Autodesk Inventor part; units mm, degrees
ref_plane "YZ Plane" through (0, 0, 0) normal (1, 0, 0) x (0, 1, 0)
ref_plane "XZ Plane" through (0, 0, 0) normal (0, 1, 0) x (-1, 0, 0)
ref_plane "XY Plane" through (0, 0, 0) normal (0, 0, 1) x (1, 0, 0)
sketch "Sketch1" plane through (0, 0, 0) normal (0, 1, 0) x (-1, 0, 0)
  line L0 (85, -50) -> (65, -50)
  line L1 (-85, -50) -> (-85, 0)
  line L2 (-85, 0) -> (85, 0)
  line L3 (85, 0) -> (85, -50)
  line L4 (85, -50) -> (-85, 0) construction
  line L5 (-85, -50) -> (85, 0) construction
  arc A0 (65, -50) -> (-65, -50) centre (0, -126.0208) ccw
  line L6 (65, -50) -> (-65, -50) construction
  line L7 (-65, -50) -> (-85, -50)
  line L8 (65, -28.5948) -> (65, -14)
  line L9 (63, -12) -> (30.2021, -12)
  arc A1 (61.914, -30.2742) -> (29.6815, -15.931) centre (0, -126.0208) ccw
  line L10 (0, 0) -> (0, -25)
  arc A2 (30.2021, -12) -> (29.6815, -15.931) centre (30.2021, -14) ccw
  arc A3 (65, -14) -> (63, -12) centre (63, -14) ccw
  arc A4 (61.914, -30.2742) -> (65, -28.5948) centre (63, -28.5948) ccw
  line L11 (-65, -28.5948) -> (-65, -14)
  line L12 (-63, -12) -> (-30.2021, -12)
  arc A5 (-29.6815, -15.931) -> (-61.914, -30.2742) centre (0, -126.0208) ccw
  arc A6 (-29.6815, -15.931) -> (-30.2021, -12) centre (-30.2021, -14) ccw
  arc A7 (-63, -12) -> (-65, -14) centre (-63, -14) ccw
  arc A8 (-65, -28.5948) -> (-61.914, -30.2742) centre (-63, -28.5948) ccw
  point P0 (0, -25)
  point P1 (0, -25)
  point P2 (65, -32.3419)
  point P3 (0, -12)
  dimension "d0" = 170
  dimension "d1" = 50
  dimension "d2" = 26
  dimension "d3" = 20
  dimension "d4" = 12
  dimension "d5" = 20
  dimension "d6" = 2
extrude "Extrusion1" add sketch "Sketch1" along normal mid plane 3.175
sketch "Sketch2" plane through (0, 1.5875, 0) normal (0, 1, 0) x (1, 0, 0)
  line L0 (-85, 0) -> (85, 0)
  line L1 (-85, 50) -> (-85, 0)
  line L2 (-65, 50) -> (-85, 50)
  line L3 (0, 0) -> (0, 15.0505)
  point P0 (-75, 10)
  point P1 (-75, 40)
  point P2 (75, 10)
  point P3 (75, 40)
  dimension "d9" = 10
  dimension "d10" = 10
  dimension "d11" = 10
hole "Hole1" at (-75, 1.5875, -10) at (75, 1.5875, -10) direction (0, -1, 0) diameter 5 end through all
sketch "Sketch5" plane through (0, 1.5875, 0) normal (0, 1, 0) x (1, 0, 0)
  line L0 (-85, 0) -> (85, 0)
  point P0 (0, 0)
  point P1 (0, 7)
  point P2 (0, 19)
  point P3 (0, 0)
  dimension "d38" = 7
  dimension "d39" = 19
hole "Hole4" at (0, 1.5875, -7) at (0, 1.5875, -19) direction (0, -1, 0) diameter 5.5 end through all
sketch "Sketch6" plane through (0, -1.5875, 0) normal (0, -1, 0) x (1, 0, 0)
  line L0 (73, -10) -> (77, -10) construction
  circle A0 centre (75, -10) radius 2.5
  line L1 (73, -12.5) -> (77, -12.5)
  line L2 (77, -7.5) -> (73, -7.5)
  arc A1 (73, -7.5) -> (73, -12.5) centre (73, -10) ccw
  arc A2 (77, -12.5) -> (77, -7.5) centre (77, -10) ccw
  point P0 (0, 0)
  dimension "d47" = 4
extrude "Extrusion2" cut sketch "Sketch6" against normal blind 25.4
properties part number "Y-Axis_Cross_Bracket_LM3043" material "Aluminum 6061"
Work out the finished part from the listing and answer in its coordinate system (mm). A direction names the side the tool comes from. Give positions to 0.01 mm unless a question says otherwise; leave off trailing zeros. Write each loop counter-clockwise with the first axis right and the second up, starting at its lowest first coordinate (ties: lowest second). Pieces come first, ordered by that corner, then holes.
(1) The part is cut by section A-A on x = 0. Write down the section's boundary in (y, z), plus the area to 3 significant figures.
Final values:
outline: (-1.59, -26) - (1.59, -26) - (1.59, -21.75) - (-1.59, -21.75) - close; (-1.59, -16.25) - (1.59, -16.25) - (1.59, -9.75) - (-1.59, -9.75) - close; (-1.59, -4.25) - (1.59, -4.25) - (1.59, 0) - (-1.59, 0) - close
area: 47.6 mm2
(2) Which of the six approach directions +Z, -Z, +X, -X, +Y, -Y give full straight-line access (tool end or side, diameter ignored) to faces 5 (the flat face through (-65, 0, -21)), 6 (the cylindrical face through (0.991, -0.022, -26.005))?
Final values:
face 5: +Y, -Y
face 6: -Z, +Y, -Y
(3) The part is cut by section D-D on x = -75. Write down the section's boundary in (y, z), plus the area to 3 significant figures.
Final values:
outline: (-1.59, -50) - (1.59, -50) - (1.59, -12.5) - (-1.59, -12.5) - close; (-1.59, -7.5) - (1.59, -7.5) - (1.59, 0) - (-1.59, 0) - close
area: 143 mm2
(4) Flat-ended cylindrical pins translate along their axes: pin 1 Ø3.5 at (x, z) = (0, -7) entering from +Y; pin 2 Ø1 at (x, y) = (-25.5, 0.5) entering from +Z; pin 3 Ø1 at (x, y) = (53, -0.5) entering from -Z. Find the tip coordinate at first contact, or state that the pin passes through.
Final values:
pin 1: passes through
pin 2: stops at z = 0
pin 3: stops at z = -41.51
(5) The mould has two halves that part along Z. Classify faces 1 (the flat face through (1, 0, 0)), 2 (the cylindrical face through (70.5, 0, -9.9)), 3 (the flat face through (85, 0, -25)), 4 (the flat face through (75, 0, -50)): pulls with the +Z half, pulls with the -Z half, needs draft (parallel to the pull), parting line crosses it, or undercut.
Final values:
face 1: pulls with the +Z half
face 2: undercut
face 3: needs draft
face 4: pulls with the -Z half
(6) The part is cut by section B-B on y = 1. Write down the section's boundary in (x, z), plus the area to 3 significant figures.
Final values:
outline: (-85, -50) - (-65, -50) arc R100.02 cw to (65, -50) - (85, -50) - (85, 0) - (-85, 0) - close; hole circle Ø5 at (-75, -10); hole (-65, -28.59) arc R2 ccw to (-61.91, -30.27) arc R114.02 cw to (-29.68, -15.93) arc R2 ccw to (-30.2, -12) - (-63, -12) arc R2 ccw to (-65, -14) - close; hole circle Ø5.5 at (0, -19); hole circle Ø5.5 at (0, -7); hole (29.68, -15.93) arc R114.02 cw to (61.91, -30.27) arc R2 ccw to (65, -28.59) - (65, -14) arc R2 ccw to (63, -12) - (30.2, -12) arc R2 ccw to start; hole (73, -12.5) - (77, -12.5) arc R2.5 ccw to (77, -7.5) - (73, -7.5) arc R2.5 ccw to start
area: 5,490 mm2
(7) The part is cut by section C-C on z = -18. Write down the section's boundary in (x, y), plus the area to 3 significant figures.
Final values:
outline: (-85, -1.59) - (-65, -1.59) - (-65, 1.59) - (-85, 1.59) - close; (-36.5, -1.59) - (-2.56, -1.59) - (-2.56, 1.59) - (-36.5, 1.59) - close; (2.56, -1.59) - (36.5, -1.59) - (36.5, 1.59) - (2.56, 1.59) - close; (65, -1.59) - (85, -1.59) - (85, 1.59) - (65, 1.59) - close
area: 343 mm2
(8) Straight lines are drawn through the part: line 1 (X direction, y = -0.25, z = -10); line 2 (X direction, y = 0, z = -7); line 3 (Z direction, x = -75, y = -0.35). For each, find the intervals that lie inside material, in ascending order.
Final values:
line 1: x = -85 to -77.5, -72.5 to 70.5, 79.5 to 85
line 2: x = -85 to -2.75, 2.75 to 85
line 3: z = -50 to -12.5, -7.5 to 0
